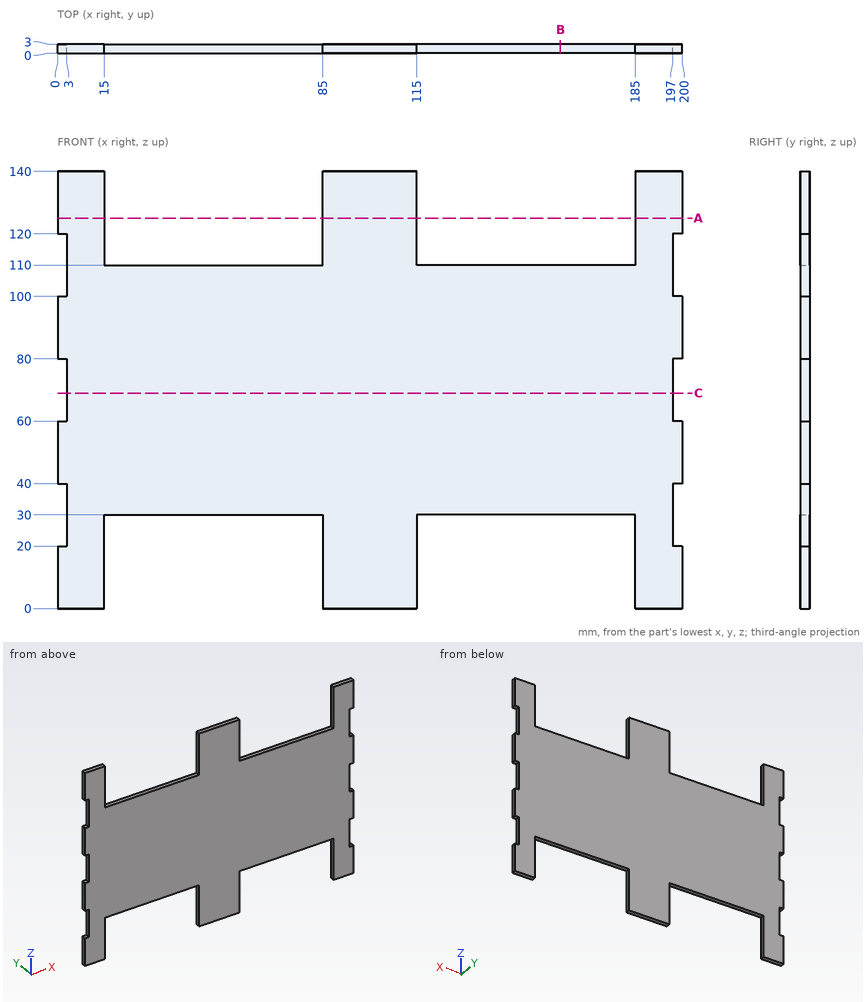
Design review of the part shown in the three views and the two pictorial views. Dimensions are in mm from the part's minimum x, y and z. Coordinates: 2 decimals unless noted, no trailing zeros. Loops run counter-clockwise (first coordinate to the right, second up) from the corner with the lowest first, then second, coordinate; pieces in that order, holes last.
(1) Wall thickness on L1, parallel to X at y = 2.85, z = 7; L2, parallel to X at y = 1.4, z = 29; L3, parallel to X at y = 1.05, z = 33.5: over which ranges is each line inside the solid? List them lowest first.
Determined:
L1: x = 0 to 15, 85 to 115, 185 to 200
L2: x = 3 to 15, 85 to 115, 185 to 197
L3: x = 3 to 197
(2) Consider section B-B, the plane x = 161. Give the boundary of the cut face in (y, z), plus the area to 3 significant figures.
Determined:
outline: (0, 30) - (3, 30) - (3, 110) - (0, 110) - close
area: 240 mm2
(3) Insertion check: P1, Ø0.9, axis at y = 2, z = 70, coming from the -X side. The pin has a flat end and moves straight along its axis. Give the tip position at first contact, or say it passes through.
Determined:
P1: stops at x = 3
(4) Consider section A-A, the plane z = 125. Give the boundary of the cut face in (x, y).
Determined:
outline: (0, 0) - (15, 0) - (15, 3) - (0, 3) - close; (85, 0) - (115, 0) - (115, 3) - (85, 3) - close; (185, 0) - (200, 0) - (200, 3) - (185, 3) - close
(5) Consider section C-C, the plane z = 69. Give the boundary of the cut face in (x, y), plus the area to 3 significant figures.
Determined:
outline: (3, 0) - (197, 0) - (197, 3) - (3, 3) - close
area: 582 mm2
